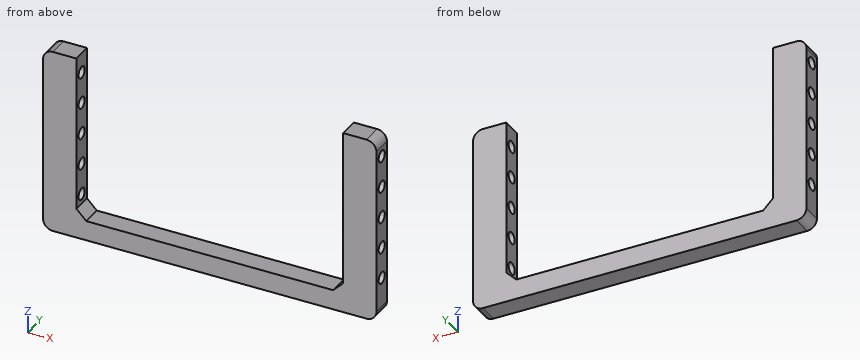
from build123d import *

# Parameters (mm, degrees)
BOSS_EXTRUDE1_DEPTH     = 3
SKETCH2_R               = 0.875
CUT_EXTRUDE1_DEPTH      = 51
CUT_EXTRUDE1_DEPTH_BACK = 3
FILLET2_R               = 1.5
CHAMFER1_SIZE           = 1.5


with BuildPart() as part:
    # Sketch1 → Boss-Extrude1 (new body)
    with BuildSketch(Plane(origin=(0, 0, 0), x_dir=(1, 0, 0), z_dir=(0, 1, 0))):
        Polygon((-25, -14), (-20, -14), (-20, 11), (20, 11), (20, -14), (25, -14), (25, 14), (-25, 14), align=None)
    extrude(amount=BOSS_EXTRUDE1_DEPTH)

    # Sketch2 → Cut-Extrude1 (cut, two sides)
    with BuildSketch(Plane.ZY.offset(-25)) as cut_extrude1_sk:
        with Locations((11, 1.5)):
            Circle(SKETCH2_R)
        with Locations((6.25, 1.5)):
            Circle(SKETCH2_R)
        with Locations((1.5, 1.5)):
            Circle(SKETCH2_R)
        with Locations((-3.25, 1.5)):
            Circle(SKETCH2_R)
        with Locations((-8, 1.5)):
            Circle(SKETCH2_R)
    extrude(amount=CUT_EXTRUDE1_DEPTH, mode=Mode.SUBTRACT)
    extrude(cut_extrude1_sk.sketch, amount=-CUT_EXTRUDE1_DEPTH_BACK, mode=Mode.SUBTRACT)

    # Fillet2
    fillet2_edges = [part.edges().sort_by_distance(p)[0] for p in [
        (25, 1.5, 14),
        (-25, 1.5, 14),
        (-25, 1.5, -14),
        (25, 1.5, -14),
    ]]
    fillet(fillet2_edges, radius=FILLET2_R)

    # Chamfer1
    chamfer1_edges = [part.edges().sort_by_distance(p)[0] for p in [
        (20, 1.5, -11),
        (-20, 1.5, -11),
    ]]
    chamfer(chamfer1_edges, length=CHAMFER1_SIZE)


solid = part.part
The model under review builds one solid part; all positions refer to its coordinate system, in mm. Round coordinates to 2 decimals unless told otherwise and drop trailing zeros. Loops run counter-clockwise (first coordinate to the right, second up) from the corner with the lowest first, then second, coordinate; pieces in that order, holes last. Notation, with made-up numbers: (44.5, -39.75) -> (78.5, -39.75) arc R20 cw to (78.5, -30.75) -> close; hole circle Ø8 at (83, 66.25). An arc over 180 degrees is marked (long way). Write item = value, one per line. Start each with the question number.
Item 1: Take a section at B-B on y = 1.5. Count the separate pieces of the cut face and the enclosed holes in it, plus the area to 3 significant figures.
Item 2: Take a section at D-D on z = 1.75. Give the boundary of the cut face in (x, y), plus the area to 3 significant figures.
Item 3: Insertion check: pin 1 (1.6 mm diameter, centred on y = 1.5, z = 11, fed in from -X). The pin has a flat end and moves straight along its axis. Give the tip position at first contact, or say it passes through.
Item 4: To check wall thickness, follow L1, parallel to Z at x = -21.85, y = 1.5 (3 decimals); L2, parallel to X at y = 2.7, z = -1; L3, parallel to Y at x = -22.15, z = -8 (3 decimals). State the ranges of each line that lie inside material, in increasing order.
Item 5: Take a section at C-C on x = 19. Give the boundary of the cut face in (y, z), plus the area to 3 significant figures.
Item 6: Take a section at A-A on z = -3.25. Give the boundary of the cut face in (x, y) (3 decimals).
Result:
q1.separate_pieces = 11
q1.enclosed_holes = 0
q1.area = 313 mm²
q2.outline = (-25, 0) -> (-20, 0) -> (-20, 0.66) -> (-25, 0.66) -> close; (-25, 2.34) -> (-20, 2.34) -> (-20, 3) -> (-25, 3) -> close; (20, 0) -> (25, 0) -> (25, 0.66) -> (20, 0.66) -> close; (20, 2.34) -> (25, 2.34) -> (25, 3) -> (20, 3) -> close
q2.area = 13.2 mm²
q3.pin_1 = through
q4.L1 = -14 to -8.875, -7.125 to -4.125, -2.375 to 0.625, 2.375 to 5.375, 7.125 to 10.125, 11.875 to 14
q4.L2 = -25 to -20, 20 to 25
q4.L3 = 0 to 0.625, 2.375 to 3
q5.outline = (0, -14) -> (3, -14) -> (3, -10.5) -> (0, -10.5) -> close
q5.area = 10.5 mm²
q6.outline = (-25, 0) -> (-20, 0) -> (-20, 0.625) -> (-25, 0.625) -> close; (-25, 2.375) -> (-20, 2.375) -> (-20, 3) -> (-25, 3) -> close; (20, 0) -> (25, 0) -> (25, 0.625) -> (20, 0.625) -> close; (20, 2.375) -> (25, 2.375) -> (25, 3) -> (20, 3) -> close
